Could you check a few things on this model? Use its own coordinates, in mm. A direction names the side the tool comes from. Round coordinates to 2 decimals unless told otherwise and drop trailing zeros. Write each loop counter-clockwise with the first axis right and the second up, starting at its lowest first coordinate (ties: lowest second). Pieces come first, ordered by that corner, then holes.
Autodesk Inventor part; units mm, degrees
ref_plane "YZ Plane" through (0, 0, 0) normal (1, 0, 0) x (0, 1, 0)
ref_plane "XZ Plane" through (0, 0, 0) normal (0, 1, 0) x (-1, 0, 0)
ref_plane "XY Plane" through (0, 0, 0) normal (0, 0, 1) x (1, 0, 0)
sketch "Sketch1" plane through (0, 0, 0) normal (0, 0, 1) x (1, 0, 0)
  line L0 (0, 0) -> (8.7313, 0) construction
  line L1 (0, 0) -> (0, 7.9375) construction
  line L2 (0, 7.9375) -> (8.7312, 7.9375) construction
  line L3 (8.7312, 7.9375) -> (8.7313, 0) construction
  line L4 (8.7312, 7.9375) -> (45.2438, 7.9375) construction
  line L5 (8.7312, 7.9375) -> (8.7312, 14.2875) construction
  line L6 (8.7312, 14.2875) -> (9.525, 14.2875) construction
  line L7 (9.525, 14.2875) -> (9.525, 0) construction
  line L8 (9.525, 0) -> (8.7313, 0) construction
  line L9 (9.525, 0) -> (19.05, 0) construction
  line L10 (19.05, 0) -> (19.05, 26.67) construction
  line L11 (19.05, 26.67) -> (9.525, 26.67) construction
  line L12 (9.525, 26.67) -> (9.525, 14.2875) construction
  line L13 (14.2875, 0) -> (14.2875, 26.67) construction
  line L14 (14.2875, 17.4625) -> (21.4312, 17.4625) construction
  line L15 (21.4312, 17.4625) -> (21.4313, 0) construction
  line L16 (21.4313, 0) -> (19.05, 0) construction
  line L17 (21.4313, 0) -> (22.225, 0) construction
  line L18 (22.225, 0) -> (22.225, 14.2875) construction
  line L19 (22.225, 14.2875) -> (21.4313, 14.2875) construction
  line L20 (21.4313, 14.2875) -> (21.4313, 0) construction
  line L21 (22.225, 0) -> (31.75, 0) construction
  line L22 (31.75, 0) -> (31.75, 20.32) construction
  line L23 (31.75, 20.32) -> (22.225, 20.32) construction
  line L24 (22.225, 20.32) -> (22.225, 0) construction
  line L25 (26.9875, 20.32) -> (26.9875, 0) construction
  line L26 (26.9875, 17.4625) -> (34.1313, 17.4625) construction
  line L27 (34.1313, 17.4625) -> (34.1313, 0) construction
  line L28 (34.1313, 0) -> (31.75, 0) construction
  line L29 (34.1313, 0) -> (34.925, 0) construction
  line L30 (34.925, 0) -> (34.925, 14.2875) construction
  line L31 (34.925, 14.2875) -> (34.1313, 14.2875) construction
  line L32 (34.1313, 14.2875) -> (34.1313, 0) construction
  line L33 (34.925, 0) -> (36.5125, 0) construction
  line L34 (36.5125, 0) -> (36.5125, 9.525) construction
  line L35 (36.5125, 9.525) -> (34.925, 9.525) construction
  line L36 (34.925, 9.525) -> (34.925, 0) construction
  line L37 (45.2438, 7.9375) -> (45.2438, 0) construction
  line L38 (45.2438, 0) -> (36.5125, 0) construction
  line L39 (11.9063, 26.67) -> (11.9063, 0) construction
  line L40 (24.6063, 20.32) -> (24.6063, 0) construction
  line L41 (0, 7.9375) -> (0, 17.4625) construction
  line L42 (0, 17.4625) -> (8.7312, 17.4625) construction
  line L43 (8.7312, 17.4625) -> (8.7312, 14.2875) construction
  line L44 (0, 3.175) -> (45.2438, 3.175) construction
  circle A0 centre (11.9063, 5.5562) radius 2.3813 construction
  circle A1 centre (24.6063, 5.5562) radius 2.3812 construction
  circle A2 centre (11.9063, 5.8103) radius 2.3813 construction
  circle A3 centre (11.9063, 7.5565) radius 2.3813 construction
  circle A4 centre (24.6063, 5.8103) radius 2.3812 construction
  circle A5 centre (24.6063, 7.5565) radius 2.3812 construction
  line L45 (9.525, 8.1915) -> (14.2875, 8.1915) construction
  line L46 (12.6386, 3.175) -> (14.6388, 5.1753) construction
  line L47 (14.6388, 5.1753) -> (21.8737, 5.1753) construction
  line L48 (21.8737, 5.1753) -> (23.8739, 3.175) construction
  line L49 (22.225, 8.1915) -> (26.9875, 8.1915) construction
  line L50 (10.3187, 5.1753) -> (17.4901, 5.1753) construction
  line L51 (26.1938, 5.1753) -> (19.0224, 5.1753) construction
  line L52 (0, 6.35) -> (6.731, 6.35) construction
  line L53 (6.731, 6.35) -> (6.731, 0) construction
  line L54 (10.3187, 5.1753) -> (8.3185, 3.175) construction
  line L55 (17.4901, 5.1753) -> (19.4903, 3.175) construction
  line L56 (19.4903, 3.175) -> (26.1938, 3.175) construction
  line L57 (26.1938, 3.175) -> (28.1015, 0) construction
  line L58 (26.1938, 5.1753) -> (28.194, 3.175) construction
  line L59 (28.194, 3.175) -> (34.8974, 3.175) construction
  line L60 (34.8974, 3.175) -> (36.8052, 0) construction
  line L61 (6.731, 5.5562) -> (45.2438, 5.5563) construction
  line L62 (37.202, 0) -> (33.8635, 5.5563) construction
  line L63 (19.0224, 5.1753) -> (17.0222, 3.175) construction
  line L64 (17.0222, 3.175) -> (-3.175, 3.175) construction
  line L65 (45.2438, 7.9375) -> (45.2438, 17.4625) construction
  line L66 (45.2438, 17.4625) -> (36.5125, 17.4625) construction
  line L67 (36.5125, 17.4625) -> (36.5125, 9.525) construction
  line L68 (45.2438, 7.9375) -> (51.5938, 7.9375) construction
  line L69 (51.5938, 7.9375) -> (51.5938, 0) construction
  line L70 (51.5938, 0) -> (45.2438, 0) construction
  line L71 (51.5938, 6.35) -> (64.2938, 6.35) construction
  line L72 (64.2938, 6.35) -> (64.2938, 0) construction
  line L73 (64.2938, 0) -> (51.5938, 0) construction
  line L74 (-8.1534, 3.175) -> (-8.1534, 2.3812) construction
  line L75 (-8.1534, 0) -> (36.8052, 0) construction
  line L76 (-3.175, 3.175) -> (-3.175, 2.3812) construction
  line L77 (-3.175, 2.3812) -> (-8.1534, 2.3812) construction
  line L78 (-8.1534, 3.175) -> (-8.1534, 6.35) construction
  line L79 (-8.1534, 6.35) -> (-3.175, 6.35) construction
  line L80 (-3.175, 6.35) -> (-3.175, 3.175) construction
  line L81 (-3.175, 0) -> (-3.175, 2.3812) construction
  line L82 (-0.7937, 0) -> (-0.7938, 11.1125) construction
  line L83 (-0.7938, 11.1125) -> (-3.175, 11.1125) construction
  line L84 (-3.175, 11.1125) -> (-3.175, 6.35) construction
  line L85 (-3.175, 3.175) -> (-8.1534, 3.175) construction
  line L86 (-8.1534, 2.3812) -> (-8.1534, 0) construction
  line L87 (-8.1534, 2.7051) -> (-9.652, 2.7051) construction
  line L88 (-9.652, 2.7051) -> (-9.652, 0) construction
  line L89 (-9.652, 0) -> (-8.1534, 0) construction
  line L90 (-8.1534, 1.4224) -> (-5.6134, 1.4224) construction
  line L91 (-5.6134, 1.4224) -> (-5.6134, 0) construction
  line L92 (-5.6134, 1.4224) -> (-3.0734, 1.4224) construction
  line L93 (-3.0734, 1.4224) -> (-3.0734, 0) construction
  line L94 (-3.175, 11.1125) -> (-13.4938, 11.1125) construction
  line L95 (-13.4938, 11.1125) -> (-13.4937, 5.9531) construction
  line L96 (-13.4937, 5.9531) -> (-18.5801, 5.9531) construction
  line L97 (-18.5801, 5.9531) -> (-18.5801, 0) construction
  line L98 (-18.5801, 0) -> (-9.652, 0) construction
  line L99 (-8.1534, 3.9687) -> (-14.6113, 3.9687) construction
  line L100 (-14.6113, 3.9687) -> (-14.6113, 0) construction
  line L101 (-14.6113, 3.429) -> (-10.4457, 3.429) construction
  line L102 (-10.4457, 3.429) -> (-10.4457, 0) construction
  line L103 (-16.9926, 3.175) -> (-16.9926, 0) construction
  line L104 (-16.9926, 3.175) -> (-18.5801, 3.175) construction
  dimension "d0" = 8.7312
  dimension "d1" = 7.9375
  dimension "d2" = 0.7937
  dimension "d3" = 14.2875
  dimension "d4" = 9.525
  dimension "d5" = 26.67
  dimension "d6" = 7.1437
  dimension "d7" = 17.4625
  dimension "d8" = 0.7937
  dimension "d9" = 14.2875
  dimension "d10" = 9.525
  dimension "d11" = 20.32
  dimension "d12" = 7.1437
  dimension "d13" = 17.4625
  dimension "d14" = 0.7937
  dimension "d15" = 14.2875
  dimension "d16" = 1.5875
  dimension "d17" = 9.525
  dimension "d18" = 8.7312
  dimension "d19" = 2.3813
  dimension "d20" = 2.3813
  dimension "d21" = 17.4625
  dimension "d22" = 3.175
  dimension "d23" = 4.7625
  dimension "d24" = 4.7625
  dimension "d26" = 0.254
  dimension "d28" = 45
  dimension "d29" = 45
  dimension "d30" = 0.254
  dimension "d31" = 7.2348
  dimension "d32" = 5.1753
  dimension "d33" = 7.1713
  dimension "d34" = 1.5875
  dimension "d35" = 7.1713
  dimension "d36" = 1.5875
  dimension "d37" = 6.35
  dimension "d39" = 45
  dimension "d40" = 45
  dimension "d41" = 1.5875
  dimension "d42" = 59
  dimension "d43" = 6.7034
  dimension "d44" = 6.7034
  dimension "d45" = 5.5563
  dimension "d46" = 0.3969
  dimension "d47" = 1.5875
  dimension "d48" = 6.731
  dimension "d52" = 17.4625
  dimension "d53" = 6.35
  dimension "d54" = 12.7
  dimension "d55" = 6.35
  dimension "d56" = 2.3813
  dimension "d57" = 4.9784
  dimension "d58" = 6.35
  dimension "d66" = 2.3813
  dimension "d67" = 0.7937
  dimension "d68" = 11.1125
  dimension "d69" = 2.7051
  dimension "d70" = 1.4986
  dimension "d71" = 1.4224
  dimension "d72" = 2.54
  dimension "d73" = 2.54
  dimension "d74" = 3.9688
  dimension "d75" = 4.1656
  dimension "d76" = 3.429
sketch "Sketch2" plane through (0, 0, 0) normal (0, 0, 1) x (1, 0, 0)
  line L0 (-3.175, 11.1125) -> (-3.175, 6.35)
  line L1 (-8.1534, 6.35) -> (-3.175, 6.35)
  line L2 (-8.1534, 3.9687) -> (-14.6113, 3.9687)
  line L3 (-14.6113, 3.9687) -> (-14.6113, 0)
  line L4 (-16.9926, 3.175) -> (-16.9926, 0)
  line L5 (-16.9926, 3.175) -> (-18.5801, 3.175)
  line L6 (-13.4937, 5.9531) -> (-18.5801, 5.9531)
  line L7 (-13.4938, 11.1125) -> (-13.4937, 5.9531)
  line L8 (-3.175, 11.1125) -> (-13.4938, 11.1125)
  line L9 (-18.5801, 5.9531) -> (-18.5801, 3.175)
  line L10 (-16.9926, 0) -> (-14.6113, 0)
  line L11 (-8.1534, 3.9687) -> (-8.1534, 6.35)
  point P0 (0, 0)
revolve "Revolution1" add sketch "Sketch2" angle 360 about axis through (-16.9926, 0, 0) along (1, 0, 0)
sketch "Sketch3" plane through (-16.9926, 0, 0) normal (-1, 0, 0) x (0, 0, 1)
  circle A0 centre (0, 0) radius 3.175
hole "Hole1" at (-16.9926, 0, 0) direction (1, 0, 0) diameter 4.318 end through all
sketch "Sketch5" plane through (-3.175, 0, 0) normal (1, 0, 0) x (0, 0, -1)
  circle A0 centre (0, 0) radius 6.35
  circle A1 centre (0, 0) radius 11.1125
  line L0 (-11.1125, 0) -> (-6.35, 0)
  line L1 (-6.35, 0) -> (6.35, 0)
  line L2 (6.35, 0) -> (11.1125, 0)
  circle A2 centre (-8.4074, 0) radius 2.7051
  point P0 (8.4074, 0)
  point P1 (-5.7023, 0)
  dimension "d98" = 5.4102
  dimension "d99" = 0.6477
  dimension "d100" = 2.0574
  dimension "d101" = 2.0574
hole "Hole3" at (-3.175, 0, 8.4074) at (-3.175, 0, -8.4074) direction (-1, 0, 0) diameter 2.159 depth 5.08 tip angle 118
chamfer "Chamfer1" distance 1.5875 angle 45 1 edges at (-13.4937, -11.1125, 0)
equation "\"d9\" = d3"
equation "\"d12\" = d6"
equation "\"d13\" = d7"
equation "\"d15\" = d9"
equation "\"d18\" = d0"
equation "\"d20\" = d19"
equation "\"d35\" = d33"
equation "\"d36\" = d34"
equation "\"d43\" = d44"
equation "\"d52\" = d13"
properties part number "Ball Shifting Outline" material "Aluminum 6061"
Q1. We'd pull the mould along Z, two halves only. Please class faces 4 (the conical face through (-13.494, 5.891, -1.855)), 5 (the cylindrical face through (-7.6, 10.6, -3.34)), 6 (the flat face through (-8.153, -3, -3)): pulls with the +Z half, pulls with the -Z half, needs draft (parallel to the pull), parting line crosses it, or undercut.
Q2. On a 3-axis mill with a long thin cutter (end or side, diameter ignored), from which of +Z, -Z, +X, -X, +Y, -Y can I reach the whole of each face in a straight line? I mean faces 1 (the flat face through (-3.175, 5, -5)), 2 (the flat face through (-14.611, 2, -2)), 3 (the cylindrical face through (-17.8, -0.69, 3.1)). Say none if no direction works.
Q3. If I drill on L1, parallel to Z at x = -4.3, y = 0; L2, parallel to X at y = 2, z = 6.75 (3 decimals); L3, parallel to Z at x = -9, y = -0.25, over which ranges is the centre line in solid material (lowest first)?
Q4. Imagine slicing it at C-C, the plane x = -16.25. Write out the boundary of the cut face in (y, z), then the cut area to 3 significant figures.
Q5. I'm going to push flat-ended pins straight in: pin 1 Ø2.5 at (y, z) = (1, 1) entering from +X; pin 2 Ø3 at (y, z) = (0, -8.41) entering from -X; pin 3 Ø3 at (x, z) = (-14, -8.5) entering from -Y. Where does each tip first touch, or does it pass through?
Q6. Imagine slicing it at B-B, the plane x = -7.5. Count the separate pieces of the cut face and the enclosed holes in it, then the cut area to 3 significant figures.
Q7. Imagine slicing it at A-A, the plane x = -14.25. Write out the boundary of the cut face in (y, z).
Results found:
1. face 4: needs draft
1. face 5: parting line crosses it
1. face 6: undercut
2. face 1: +Z, -Z, +X, +Y, -Y
2. face 2: +X
2. face 3: -X
3. L1: z = -11.11 to -9.49, -7.33 to -6.35, 6.35 to 7.33, 9.49 to 11.11
3. L2: x = -13.494 to -3.175
3. L3: z = -11.11 to -3.96, 3.96 to 11.11
4. outline: circle Ø11.91 at (0, 0); hole circle Ø4.32 at (0, 0)
4. area: 96.7 mm2
5. pin 1: stops at x = -14.61
5. pin 2: stops at x = -13.49
5. pin 3: stops at y = -6.83
6. separate pieces: 1
6. enclosed holes: 3
6. area: 254 mm2
7. outline: circle Ø11.91 at (0, 0); hole circle Ø7.94 at (0, 0)
